Design review of the part shown in the three views and the two pictorial views. Dimensions are in mm from the part's minimum x, y and z. Round coordinates to 2 decimals unless told otherwise and drop trailing zeros. Order: outer loops, then holes, each group sorted by start corner. A loop starts at its lowest first (then second) coordinate and runs counter-clockwise, first axis right, second up.
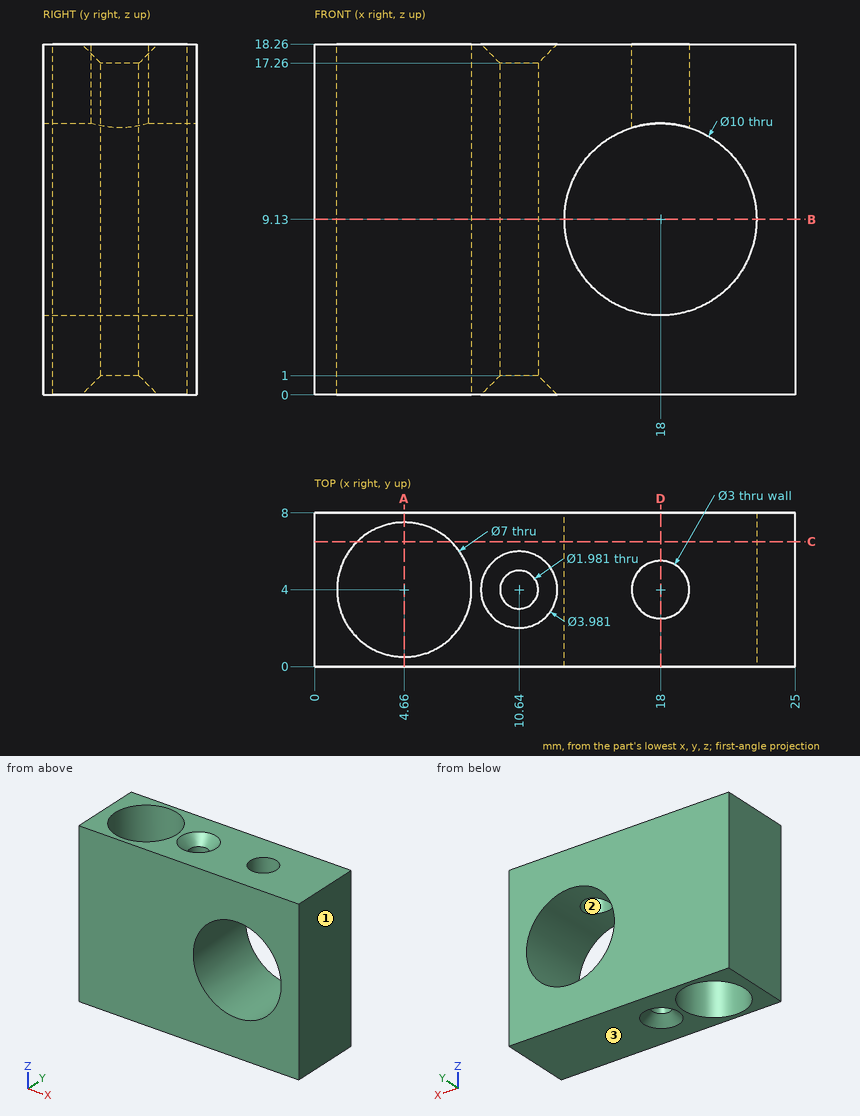
1) Take a section at B-B on z = 9.13. Give the boundary of the cut face in (x, y).
Results:
outline: (0, 0) - (13, 0) - (13, 8) - (0, 8) - close; (23, 0) - (25, 0) - (25, 8) - (23, 8) - close; hole circle Ø7 at (4.66, 4); hole circle Ø1.98 at (10.64, 4)
2) To check wall thickness, follow line 1 along Y through (x, z) = (4.66, 6.25); line 2 along Y through (x, z) = (18, 16); line 3 along X through (y, z) = (3.5, 3.5). State the ranges of each line that lie inside material, in increasing order.
Results:
line 1: y = 0 to 0.5, 7.5 to 8
line 2: y = 0 to 2.5, 5.5 to 8
line 3: x = 0 to 1.2, 8.12 to 9.78, 11.5 to 25
3) Clearance check with a flat-ended pin moving along its axis: P1, Ø1.5, axis at x = 10, y = 3.5, coming from the +Z side. State where the tip first meets the part, or that it passes through.
Results:
P1: stops at z = 17.83
4) Take a section at D-D on x = 18. Give the boundary of the cut face in (y, z), plus the area to 3 significant figures.
Results:
outline: (0, 0) - (8, 0) - (8, 4.13) - (0, 4.13) - close; (0, 14.13) - (2.5, 14.13) - (2.5, 18.26) - (0, 18.26) - close; (5.5, 14.13) - (8, 14.13) - (8, 18.26) - (5.5, 18.26) - close
area: 53.7 mm2
5) Take a section at A-A on x = 4.66. Give the boundary of the cut face in (y, z).
Results:
outline: (0, 0) - (0.5, 0) - (0.5, 18.26) - (0, 18.26) - close; (7.5, 0) - (8, 0) - (8, 18.26) - (7.5, 18.26) - close
6) Take a section at C-C on y = 6.5. Give the boundary of the cut face in (x, z).
Results:
outline: (0, 0) - (2.21, 0) - (2.21, 18.26) - (0, 18.26) - close; (7.11, 0) - (25, 0) - (25, 18.26) - (7.11, 18.26) - close; hole circle Ø10 at (18, 9.13)
7) The part is to be moulded in two halves that separate along X. For the marked faces 1, 2 and 3, say which applies: released by +X, released by -X, zero draft, split by the parting line, or undercut.
Results:
face 1: released by +X
face 2: undercut
face 3: zero draft
